from build123d import *

# Parameters (mm, degrees)
SKETCH2_W           = 120
SKETCH2_H           = 120
SKETCH2_W_2         = 90
SKETCH2_H_2         = 90
BOSS_EXTRUDE1_DEPTH = 5
SKETCH3_W           = 15
SKETCH3_H           = 15
BOSS_EXTRUDE2_DEPTH = 5
SKETCH4_R           = 2.5
CUT_EXTRUDE1_DEPTH  = 86.440037453


with BuildPart() as part:
    # Sketch2 → Boss-Extrude1 (new body)
    with BuildSketch(Plane(origin=(0, 0, 0), x_dir=(1, 0, 0), z_dir=(0, 1, 0))):
        Rectangle(SKETCH2_W, SKETCH2_H)
        Rectangle(SKETCH2_W_2, SKETCH2_H_2, mode=Mode.SUBTRACT)
    extrude(amount=BOSS_EXTRUDE1_DEPTH)

    # Sketch3 → Boss-Extrude2 (add)
    with BuildSketch(Plane(origin=(0, 5, 0), x_dir=(1, 0, 0), z_dir=(0, 1, 0))):
        with Locations((52.5, 52.5)):
            Rectangle(SKETCH3_W, SKETCH3_H)
        with Locations((-52.5, 52.5)):
            Rectangle(SKETCH3_W, SKETCH3_H)
        with Locations((52.5, -52.5)):
            Rectangle(SKETCH3_W, SKETCH3_H)
        with Locations((-52.5, -52.5)):
            Rectangle(SKETCH3_W, SKETCH3_H)
    extrude(amount=BOSS_EXTRUDE2_DEPTH)

    # Sketch4 → Cut-Extrude1 (cut, through all)
    with BuildSketch(Plane(origin=(0, 10, 0), x_dir=(1, 0, 0), z_dir=(0, 1, 0))):
        with Locations(Location((-52.5, -52.5, 0), (0, 0, 270))):
            Circle(SKETCH4_R)
        with Locations(Location((-52.5, 52.5, 0), (0, 0, 270))):
            Circle(SKETCH4_R)
        with Locations(Location((52.5, 52.5, 0), (0, 0, 270))):
            Circle(SKETCH4_R)
        with Locations(Location((52.5, -52.5, 0), (0, 0, 270))):
            Circle(SKETCH4_R)
    extrude(amount=-CUT_EXTRUDE1_DEPTH, mode=Mode.SUBTRACT)


solid = part.part
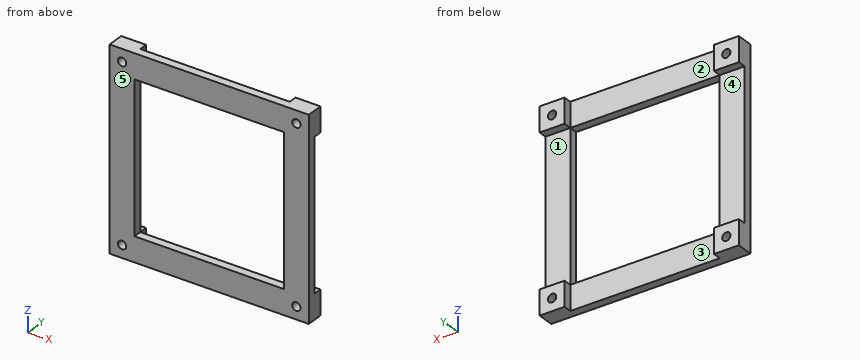
Here's how the part is built. I have some questions about the finished solid (model axes, mm). Face numbers are marked on the shaded views. A direction names the side the tool comes from. Coordinates: 2 decimals unless noted, no trailing zeros. Loops run counter-clockwise (first coordinate to the right, second up) from the corner with the lowest first, then second, coordinate; pieces in that order, holes last. Notation, with made-up numbers: (56.25, 61.25) -> (83.25, 61.25) arc R23 cw to (83.25, 99.25) -> close; hole circle Ø11 at (-28.75, -38). An arc over 180 degrees is marked (long way). Use one line per item in the form item = value. Start each with the question number.
(1) We'd pull the mould along Z, two halves only. Please class the marked faces 1 and 2: pulls with the +Z half, pulls with the -Z half, needs draft (parallel to the pull), parting line crosses it, or undercut.
(2) If we section it at A-A (x = -14): Please give me the cut outline in (y, z).
(3) If we section it at C-C (z = 2.5): Please give me the cut outline in (x, y).
(4) If we section it at B-B (y = 8.5): Please give me the cut outline in (x, z).
(5) On a 3-axis mill with a long thin cutter (end or side, diameter ignored), from which of +Z, -Z, +X, -X, +Y, -Y can I reach the whole of each face in a straight line? I mean the marked faces 3, 4 and 5. Say none if no direction works.
(6) Will these pins go through, and if not, where does the flat tip stop? pin 1 (6.5 mm diameter, centred on x = -52.5, z = 52.5, fed in from +Y); pin 2 (7.5 mm diameter, centred on x = -2.5, z = 49.5, fed in from +Y); pin 3 (4 mm diameter, centred on y = 8, z = 0.5, fed in from +X).
(7) If we section it at D-D (y = 2.5): Please give me the cut outline in (x, z), then the cut area to 3 significant figures.
(8) Please list where these lines run through material, in increasing order: line 1 along X through (y, z) = (7, -52.5); line 2 along X through (y, z) = (3.25, -52.5); line 3 along Z through (x, y) = (31, 2.5).
Verdict:
q1.face_1 = undercut
q1.face_2 = needs draft
q2.outline = (0, -60) -> (5, -60) -> (5, -45) -> (0, -45) -> close; (0, 45) -> (5, 45) -> (5, 60) -> (0, 60) -> close
q3.outline = (-60, 0) -> (-45, 0) -> (-45, 5) -> (-60, 5) -> close; (45, 0) -> (60, 0) -> (60, 5) -> (45, 5) -> close
q4.outline = (-60, -60) -> (-45, -60) -> (-45, -45) -> (-60, -45) -> close; (-60, 45) -> (-45, 45) -> (-45, 60) -> (-60, 60) -> close; (45, -60) -> (60, -60) -> (60, -45) -> (45, -45) -> close; (45, 45) -> (60, 45) -> (60, 60) -> (45, 60) -> close; hole circle Ø5 at (-52.5, -52.5); hole circle Ø5 at (-52.5, 52.5); hole circle Ø5 at (52.5, -52.5); hole circle Ø5 at (52.5, 52.5)
q5.face_3 = +Z, -Z, +Y
q5.face_4 = +X, -X, +Y
q5.face_5 = +Z, -Z, +X, -X, -Y
q6.pin_1 = 10
q6.pin_2 = 5
q6.pin_3 = through
q7.outline = (-60, -60) -> (60, -60) -> (60, 60) -> (-60, 60) -> close; hole circle Ø5 at (-52.5, -52.5); hole circle Ø5 at (-52.5, 52.5); hole (-45, -45) -> (45, -45) -> (45, 45) -> (-45, 45) -> close; hole circle Ø5 at (52.5, -52.5); hole circle Ø5 at (52.5, 52.5)
q7.area = 6,220 mm²
q8.line_1 = -60 to -55, -50 to -45, 45 to 50, 55 to 60
q8.line_2 = -60 to -55, -50 to 50, 55 to 60
q8.line_3 = -60 to -45, 45 to 60
